The model under review builds one solid part; all positions refer to its coordinate system, in mm. A direction names the side the tool comes from. Coordinates: 2 decimals unless noted, no trailing zeros. Order: outer loops, then holes, each group sorted by start corner. A loop starts at its lowest first (then second) coordinate and runs counter-clockwise, first axis right, second up. Notation, with made-up numbers: (38.5, 24) - (78.5, 24) arc R11 ccw to (78.5, 43) - close; hole circle Ø11 at (16, -23). An arc over 180 degrees is marked (long way). Answer in a Markdown table with one row per item.
```python
from build123d import *

# Parameters (mm, degrees)
SKETCH_1_W                  = 15
SKETCH_1_H                  = 15.60669
EXTRUDE_1_DEPTH             = 9
EXTRUDE_2_DEPTH             = 235
EXTRUDE_3_DEPTH             = 1
SKETCH_4_W                  = 15
SKETCH_4_H                  = 17.19706
EXTRUDE_4_DEPTH             = 10
SKETCH_5_W                  = 15
SKETCH_5_H                  = 3
CUT_EXTRUDE_1_DEPTH         = 1
SKETCH_6_W                  = 12.12351
SKETCH_6_H                  = 15
EXTRUDE_5_DEPTH             = 10
SKETCH_7_W                  = 15
SKETCH_7_H                  = 15
EXTRUDE_6_DEPTH             = 10
SKETCH_8_W                  = 15
SKETCH_8_H                  = 3
CUT_EXTRUDE_2_DEPTH         = 1
SKETCH_9_W                  = 17.81946
SKETCH_9_H                  = 15
EXTRUDE_7_DEPTH             = 10
EXTRUDE_8_DEPTH             = 15
SKETCH_11_W                 = 41.16167
SKETCH_11_H                 = 80
HOLE_WIZARD_10_0_10_1_D     = 10
HOLE_WIZARD_10_0_10_1_DEPTH = 50
HOLE_WIZARD_10_0_10_2_D     = 10
HOLE_WIZARD_10_0_10_2_DEPTH = 50
HOLE_WIZARD_4_0_4_1_D       = 4
HOLE_WIZARD_4_0_4_1_DEPTH   = 7.5
CHAMFER_1_SIZE              = 16.206633169
CHAMFER_1_EDGE_2_SIZE       = 16.206633169


with BuildPart() as part:
    # 草图1 → 凸台-拉伸1 (new body)
    with BuildSketch(Plane.XZ.offset(5)):
        with Locations((-117.5, 102.803345)):
            Rectangle(SKETCH_1_W, SKETCH_1_H)
    extrude(amount=-EXTRUDE_1_DEPTH)

    # 草图2 → 凸台-拉伸2 (add)
    with BuildSketch(Plane(origin=(-110, 0, 0), x_dir=(0, 0, -1), z_dir=(1, 0, 0))):
        Polygon((-95, 4.74906), (-95, -5), (-104.75, -5), (-104.75, -4), (-107.75, -4), (-107.75, -5), (-110, -5), (-110, 4.74906), align=None)
    extrude(amount=EXTRUDE_2_DEPTH)

    # 草图3 → 凸台-拉伸3 (add)
    with BuildSketch(Plane(origin=(0, 4, 0), x_dir=(-1, 0, 0), z_dir=(0, 1, 0))):
        Polygon((125, 95), (-125, 95), (-125, 110), (125, 110), (125, 107.75), (-110, 107.75), (-110, 104.75), (125, 104.75), align=None)
    extrude(amount=EXTRUDE_3_DEPTH)

    # 草图4 → 凸台-拉伸4 (add)
    with BuildSketch(Plane(origin=(0, 5, 0), x_dir=(-1, 0, 0), z_dir=(0, 1, 0))):
        with Locations((-117.5, 103.59853)):
            Rectangle(SKETCH_4_W, SKETCH_4_H)
    extrude(amount=EXTRUDE_4_DEPTH)

    # 草图5 → 切除-拉伸1 (cut)
    with BuildSketch(Plane.XZ.offset(-4)):
        with Locations((117.5, 106.25)):
            Rectangle(SKETCH_5_W, SKETCH_5_H)
    extrude(amount=-CUT_EXTRUDE_1_DEPTH, mode=Mode.SUBTRACT)

    # 草图6 → 凸台-拉伸5 (add)
    with BuildSketch(Plane.XZ.offset(5)):
        with Locations((116.061755, 102.5)):
            Rectangle(SKETCH_6_W, SKETCH_6_H)
    extrude(amount=EXTRUDE_5_DEPTH)

    # 草图7 → 凸台-拉伸6 (add)
    with BuildSketch(Plane.XZ.offset(5)):
        with Locations((-117.5, 102.5)):
            Rectangle(SKETCH_7_W, SKETCH_7_H)
    extrude(amount=EXTRUDE_6_DEPTH)

    # 草图8 → 切除-拉伸2 (cut)
    with BuildSketch(Plane(origin=(0, -4, 0), x_dir=(1, 0, 0), z_dir=(0, 1, 0))):
        with Locations((-117.5, -106.25)):
            Rectangle(SKETCH_8_W, SKETCH_8_H)
    extrude(amount=-CUT_EXTRUDE_2_DEPTH, mode=Mode.SUBTRACT)

    # 草图9 → 凸台-拉伸7 (add)
    with BuildSketch(Plane(origin=(0, 5, 0), x_dir=(-1, 0, 0), z_dir=(0, 1, 0))):
        with Locations((118.90973, 102.5)):
            Rectangle(SKETCH_9_W, SKETCH_9_H)
    extrude(amount=EXTRUDE_7_DEPTH)

    # 草图10 → 凸台-拉伸8 (add)
    with BuildSketch(Plane(origin=(0, 0, 95), x_dir=(-1, 0, 0), z_dir=(0, 0, -1))):
        Polygon((0, 66.136363636), (125, 15), (125, -15), (0, -66.136363636), (-125, -15), (-125, 15), align=None)
    extrude(amount=EXTRUDE_8_DEPTH)

    # 草图11 → 旋转1 (revolve)
    with BuildSketch(Plane.XZ, mode=Mode.PRIVATE) as revolve_1_sk:
        with Locations((20.580835, 40)):
            Rectangle(SKETCH_11_W, SKETCH_11_H)
    revolve(revolve_1_sk.sketch.rotate(Axis((0, 0, 80), (0, 0, -1)), 180), axis=Axis((0, 0, 80), (0, 0, -1)))

    # Ø10.0 (10) 直径孔1
    with Locations(Plane(origin=(-41.16167, 0, 10), x_dir=(0, 0, -1), z_dir=(-1, 0, 0))):
        with Locations((0, 0)):
            Hole(HOLE_WIZARD_10_0_10_1_D / 2, depth=HOLE_WIZARD_10_0_10_1_DEPTH)

    # Ø10.0 (10) 直径孔2
    with Locations(Plane(origin=(0, -41.16167, 10), x_dir=(-1, 0, 0), z_dir=(0, -1, 0))):
        with Locations((0, 0)):
            Hole(HOLE_WIZARD_10_0_10_2_D / 2, depth=HOLE_WIZARD_10_0_10_2_DEPTH)

    # Ø4.0 (4) 直径孔1
    with Locations(Plane.XY.offset(110.60669)):
        with Locations((115, 0), (69, 0), (23, 0), (-23, 0), (-69, 0), (-115, 0)):
            Hole(HOLE_WIZARD_4_0_4_1_D / 2, depth=HOLE_WIZARD_4_0_4_1_DEPTH)

    # 倒角1
    chamfer_1_edges = [part.edges().sort_by_distance(p)[0] for p in [
        (0, 66.136363636, 87.5),
    ]]
    chamfer(chamfer_1_edges, length=CHAMFER_1_SIZE)

    # 倒角1 edge 2
    chamfer_1_edge_2_edges = [part.edges().sort_by_distance(p)[0] for p in [
        (0, -66.136363636, 87.5),
    ]]
    chamfer(chamfer_1_edge_2_edges, length=CHAMFER_1_EDGE_2_SIZE)


solid = part.part
```
Item 1: We need section D-D, the plane y = 23.5. Write out the cut boundary in (x, z).
Check values:
| item | result |
|---|---|
| outline | (-104.22, 80) - (-33.79, 80) - (-33.79, 0) - (33.79, 0) - (33.79, 80) - (104.22, 80) - (104.22, 95) - (-104.22, 95) - close |
Item 2: Mouldability with a two-part tool opening along X and no side actions: class faces 4 (the face through (-70.77, -37.185, 87.605)), 5 (the face through (0, 8.838, 10)), 6 (the face through (-121, 5, 105)) as +X half, -X half, draft (parallel to the pull), parting line (faces both ways), or undercut.
Check values:
| item | result |
|---|---|
| face 4 | -X half |
| face 5 | undercut |
| face 6 | draft |
Item 3: Tool access review of faces 1 (the face through (110, 10, 103)), 2 (the face through (-118, -10, 110)), 3 (the face through (110, -10, 102)): name each direction out of +Z, -Z, +X, -X, +Y, -Y from which nothing blocks a thin tool from reaching the whole face with its end or side.
Check values:
| item | result |
|---|---|
| face 1 | +Z, +Y |
| face 2 | +Z, +X, -X, -Y |
| face 3 | +Z, -Y |
Item 4: We need section C-C, the plane z = 61. Write out the cut boundary in (x, y), then the cut area to 3 significant figures.
Check values:
| item | result |
|---|---|
| outline | circle Ø82.32 at (0, 0) |
| area | 5,320 mm^2 |
Item 5: Clearance check with flat-ended pins moving along their axes: pin 1 Ø3.5 at (x, z) = (120.5, 105.5) entering from -Y; pin 2 Ø3 at (y, z) = (-3, 58.5) entering from +X; pin 3 Ø1.2 at (x, y) = (-22.5, -0.5) entering from +Z; pin 4 Ø12 at (y, z) = (-47.5, 45) entering from +X. State where each tip first meets the part, or that it passes through.
Check values:
| item | result |
|---|---|
| pin 1 | y = -15 |
| pin 2 | x = 41.13 |
| pin 3 | z = 103.11 |
| pin 4 | through |
Item 6: We need section A-A, the plane y = -36.5. Write out the cut boundary in (x, z), then the cut area to 3 significant figures.
Check values:
| item | result |
|---|---|
| outline | (-72.44, 80) - (-19.03, 80) - (-19.03, 0) - (19.03, 0) - (19.03, 80) - (72.44, 80) - (72.44, 95) - (-72.44, 95) - close; hole circle Ø10 at (0, 10) |
| area | 5,140 mm^2 |
Item 7: To check wall thickness, follow line 1 (Y direction, x = 115, z = 105.5); line 2 (Y direction, x = -23, z = 105); line 3 (Z direction, x = -4.5, y = 39). State the ranges of each line that lie inside material, in increasing order. Write a range as from..to.
Check values:
| item | result |
|---|---|
| line 1 | -15..-5, -4..-2, 2..4, 5..15 |
| line 2 | -4..-2, 2..4.75 |
| line 3 | 0..95 |
Item 8: We need section B-B, the plane x = -64.5. Write out the cut boundary in (y, z), then the cut area to 3 significant figures.
Check values:
| item | result |
|---|---|
| outline | (-39.75, 80) - (39.75, 80) - (39.75, 95) - (5, 95) - (5, 104.75) - (4.75, 104.75) - (4.75, 107.75) - (5, 107.75) - (5, 110) - (-5, 110) - (-5, 107.75) - (-4, 107.75) - (-4, 104.75) - (-5, 104.75) - (-5, 95) - (-39.75, 95) - close |
| area | 1,340 mm^2 |
